The listing builds one solid part. Answer for the finished solid, in the listing's coordinates (mm). A direction names the side the tool comes from. Round coordinates to 2 decimals unless told otherwise and drop trailing zeros. Order: outer loops, then holes, each group sorted by start corner. A loop starts at its lowest first (then second) coordinate and runs counter-clockwise, first axis right, second up. Notation, with made-up numbers: M -5.5,-0.75 L 42.5,-0.75 A15 ccw 42.5,20.25 Z; hole C 16.5,7 d1. An arc over 180 degrees is marked long. Put each result on its own line as item: value. Start each with the question number.
1. The part is cut by section B-B (y = 28). Give the vertices of the cut face in (x, z).
2. The part is cut by section A-A (z = 2.25). Give the vertices of the cut face in (x, y), then the cut area to 3 significant figures.
3. The part is cut by section C-C (x = -28). Give the vertices of the cut face in (y, z).
4. The part is cut by section D-D (x = -52). Give the vertices of the cut face in (y, z).
5. The mould has two halves that part along Y. Classify faces 4 (the face through (-58, 22.298, 4)), 5 (the face through (-59, 28, 2.9)), 6 (the face through (-37, 33, 7.6)): +Y half, -Y half, draft (parallel to the pull), parting line (faces both ways), or undercut.
6. Consider line 1 (Y direction, x = -54, z = 4); line 2 (Z direction, x = -61, y = 33); line 3 (X direction, y = 30.5, z = 5.5). Determine where each line is inside the solid, lowest interval first.
7. Which of the six approach directions +Z, -Z, +X, -X, +Y, -Y give full straight-line access (tool end or side, diameter ignored) to faces 1 (the face through (-37, 26.648, 3)), 2 (the face through (-59, 33.498, 4)), 3 (the face through (-63, 25.848, 8))?
8. Each of these flat-tipped pins is pushed along its axis until it touches: pin 1 Ø0.9 at (y, z) = (27.5, 3.5) entering from -X; pin 2 Ø2.5 at (y, z) = (28.5, 3.5) entering from +X; pin 3 Ø7.5 at (x, y) = (-36.5, 32.5) entering from +Z. Where does it stop, or does it pass through?
from build123d import *

# Parameters (mm, degrees)
SKETCH1_W           = 39.5
SKETCH1_H           = 16.2
SKETCH1_R           = 1.5
BOSS_EXTRUDE1_DEPTH = 1.6
BOSS_EXTRUDE2_DEPTH = 6
SKETCH3_W           = 12.85
SKETCH3_H           = 3
CUT_EXTRUDE1_DEPTH  = 3
CUT_EXTRUDE3_DEPTH  = 3
SKETCH5_W           = 2.25
SKETCH5_H           = 2.25
CUT_EXTRUDE4_DEPTH  = 50.733422671
BOSS_EXTRUDE3_DEPTH = 6.75
CUT_EXTRUDE5_DEPTH  = 1.5
SKETCH8_W           = 2.65
SKETCH8_H           = 9.9
CUT_EXTRUDE6_DEPTH  = 12
CUT_EXTRUDE7_REACH  = 76.987
SKETCH9_W           = 0.35
SKETCH9_H           = 3
SKETCH9_W_2         = 0.175
BOSS_EXTRUDE4_DEPTH = 4.75
SKETCH11_W          = 12.85
SKETCH11_H          = 1.15
CUT_EXTRUDE8_DEPTH  = 4.75


with BuildPart() as part:
    # Sketch1 → Boss-Extrude1 (new body)
    with BuildSketch(Plane.XY):
        with Locations((-43.509331094, 28.548203647)):
            Rectangle(SKETCH1_W, SKETCH1_H)
        with Locations((-27.259331094, 33.648203647)):
            Circle(SKETCH1_R, mode=Mode.SUBTRACT)
        with Locations((-46.009331094, 33.648203647)):
            Circle(SKETCH1_R, mode=Mode.SUBTRACT)
    extrude(amount=BOSS_EXTRUDE1_DEPTH)

    # Sketch2 → Boss-Extrude2 (add)
    with BuildSketch(Plane.XY.offset(1.6)):
        Polygon((-30.509331094, 30.378901516), (-30.509331094, 36.648203647), (-43.359331094, 36.648203647), (-43.359331094, 26.648203647), (-30.509331094, 26.648203647), align=None)
    extrude(amount=BOSS_EXTRUDE2_DEPTH)

    # Sketch3 → Cut-Extrude1 (cut)
    with BuildSketch(Plane.XY.offset(7.6)):
        with Locations((-36.934331094, 28.148203647)):
            Rectangle(SKETCH3_W, SKETCH3_H)
    extrude(amount=-CUT_EXTRUDE1_DEPTH, mode=Mode.SUBTRACT)

    # Sketch4 → Cut-Extrude3 (cut)
    with BuildSketch(Plane.XY.offset(4.6)):
        Polygon((-32.509331094, 29.648203647), (-35.934331094, 29.648203647), (-35.934331094, 26.648203647), (-32.509331094, 26.648203647), (-32.509331094, 27.856511678), align=None)
        Polygon((-37.934331094, 29.648203647), (-41.359331094, 29.648203647), (-41.359331094, 28.148203647), (-41.359331094, 26.648203647), (-37.934331094, 26.648203647), align=None)
    extrude(amount=-CUT_EXTRUDE3_DEPTH, mode=Mode.SUBTRACT)

    # Sketch5 → Cut-Extrude4 (cut, through all)
    with BuildSketch(Plane(origin=(-30.509331094, 0, 0), x_dir=(0, 0, -1), z_dir=(1, 0, 0))):
        with Locations((-2.725, 28.523203647)):
            Rectangle(SKETCH5_W, SKETCH5_H)
    extrude(amount=-CUT_EXTRUDE4_DEPTH, mode=Mode.SUBTRACT)

    # Sketch6 → Boss-Extrude3 (add)
    with BuildSketch(Plane.XY.offset(1.6)):
        Polygon((-63.259331094, 22.298203647), (-63.259331094, 28.548203647), (-63.259331094, 34.798203647), (-65.259331094, 34.798203647), (-65.259331094, 22.298203647), align=None)
        Polygon((-63.259331094, 34.798203647), (-63.259331094, 28.548203647), (-63.259331094, 22.298203647), (-51.259331094, 22.298203647), (-51.259331094, 34.798203647), align=None)
    extrude(amount=BOSS_EXTRUDE3_DEPTH)

    # Sketch7 → Cut-Extrude5 (cut)
    with BuildSketch(Plane.XY.offset(8.35)):
        Polygon((-65.259331094, 34.798203647), (-65.259331094, 32.448203647), (-61.509331094, 32.448203647), (-61.509331094, 31.248203647), (-64.009331094, 31.248203647), (-64.009331094, 25.848203647), (-61.509331094, 25.848203647), (-61.509331094, 24.648203647), (-65.259331094, 24.648203647), (-65.259331094, 22.298203647), (-51.259331094, 22.298203647), (-51.259331094, 34.798203647), align=None)
    extrude(amount=-CUT_EXTRUDE5_DEPTH, mode=Mode.SUBTRACT)

    # Sketch8 → Cut-Extrude6 (cut)
    with BuildSketch(Plane.ZY.offset(65.259331094)):
        Polygon((6.85, 31.148203647), (5.55, 31.148203647), (5.55, 25.948203647), (6.85, 25.948203647), (7.6, 25.948203647), (7.6, 31.148203647), align=None)
        with Locations((4.225, 28.548203647)):
            Rectangle(SKETCH8_W, SKETCH8_H)
    extrude(amount=-CUT_EXTRUDE6_DEPTH, mode=Mode.SUBTRACT)

    # Cut-Extrude7: up to this face of the body (flat: up to its plane)
    cut_extrude7_end = Plane(part.part.faces().sort_by_distance((-39.983883979, 27.291998742, 1.6))[0])
    # Sketch9 → Cut-Extrude7 (cut, up to the picked face)
    with BuildSketch(Plane.XY.offset(4.6), mode=Mode.PRIVATE) as cut_extrude7_sk1:
        with Locations((-30.684331094, 28.148203647)):
            Rectangle(SKETCH9_W, SKETCH9_H)
    cut_extrude7_tool1 = split(extrude(cut_extrude7_sk1.sketch, amount=-CUT_EXTRUDE7_REACH, mode=Mode.PRIVATE), bisect_by=cut_extrude7_end, keep=Keep.BOTH, mode=Mode.PRIVATE)
    # Sketch9 → Cut-Extrude7 (cut, up to the picked face)
    with BuildSketch(Plane.XY.offset(4.6), mode=Mode.PRIVATE) as cut_extrude7_sk2:
        with Locations((-43.184331094, 28.148203647)):
            Rectangle(SKETCH9_W, SKETCH9_H)
    cut_extrude7_tool2 = split(extrude(cut_extrude7_sk2.sketch, amount=-CUT_EXTRUDE7_REACH, mode=Mode.PRIVATE), bisect_by=cut_extrude7_end, keep=Keep.BOTH, mode=Mode.PRIVATE)
    # Sketch9 → Cut-Extrude7 (cut, up to the picked face)
    with BuildSketch(Plane.XY.offset(4.6), mode=Mode.PRIVATE) as cut_extrude7_sk3:
        with Locations((-37.846831094, 28.148203647)):
            Rectangle(SKETCH9_W_2, SKETCH9_H)
    cut_extrude7_tool3 = split(extrude(cut_extrude7_sk3.sketch, amount=-CUT_EXTRUDE7_REACH, mode=Mode.PRIVATE), bisect_by=cut_extrude7_end, keep=Keep.BOTH, mode=Mode.PRIVATE)
    # Sketch9 → Cut-Extrude7 (cut, up to the picked face)
    with BuildSketch(Plane.XY.offset(4.6), mode=Mode.PRIVATE) as cut_extrude7_sk4:
        with Locations((-36.021831094, 28.148203647)):
            Rectangle(SKETCH9_W_2, SKETCH9_H)
    cut_extrude7_tool4 = split(extrude(cut_extrude7_sk4.sketch, amount=-CUT_EXTRUDE7_REACH, mode=Mode.PRIVATE), bisect_by=cut_extrude7_end, keep=Keep.BOTH, mode=Mode.PRIVATE)
    add(cut_extrude7_tool1.solids().sort_by(Axis((-30.684331, 28.148204, 4.6), (0, 0, -1)))[0], mode=Mode.SUBTRACT)
    add(cut_extrude7_tool2.solids().sort_by(Axis((-43.184331, 28.148204, 4.6), (0, 0, -1)))[0], mode=Mode.SUBTRACT)
    add(cut_extrude7_tool3.solids().sort_by(Axis((-37.846831, 28.148204, 4.6), (0, 0, -1)))[0], mode=Mode.SUBTRACT)
    add(cut_extrude7_tool4.solids().sort_by(Axis((-36.021831, 28.148204, 4.6), (0, 0, -1)))[0], mode=Mode.SUBTRACT)

    # Sketch10 → Boss-Extrude4 (add)
    with BuildSketch(Plane.XY.offset(7.6)):
        Polygon((-30.509331094, 40.033691869), (-43.359331094, 36.648203647), (-42.954120568, 36.648203647), (-30.509331094, 39.809326044), align=None)
    extrude(amount=-BOSS_EXTRUDE4_DEPTH)

    # Sketch11 → Cut-Extrude8 (cut)
    with BuildSketch(Plane(origin=(0, 36.648203647, 0), x_dir=(1, 0, 0), z_dir=(0, 1, 0))):
        with Locations((-36.934331094, -7.025)):
            Rectangle(SKETCH11_W, SKETCH11_H)
    extrude(amount=CUT_EXTRUDE8_DEPTH, mode=Mode.SUBTRACT)


solid = part.part
Resolved:
1. outline: M -65.26,1.6 L -63.26,1.6 L -63.26,0 L -23.76,0 L -23.76,1.6 L -51.26,1.6 L -51.26,6.85 L -53.26,6.85 L -53.26,2.9 L -65.26,2.9 Z; M -65.26,7.6 L -64.01,7.6 L -64.01,8.35 L -65.26,8.35 Z; M -43.01,3.85 L -41.36,3.85 L -41.36,4.6 L -43.01,4.6 Z; M -37.76,3.85 L -36.11,3.85 L -36.11,4.6 L -37.76,4.6 Z; M -32.51,3.85 L -30.86,3.85 L -30.86,4.6 L -32.51,4.6 Z
2. outline: M -65.26,22.3 L -51.26,22.3 L -51.26,34.8 L -65.26,34.8 Z; M -43.36,29.65 L -30.51,29.65 L -30.51,36.65 L -43.36,36.65 Z; M -43.01,26.65 L -41.36,26.65 L -41.36,27.4 L -43.01,27.4 Z; M -37.76,26.65 L -36.11,26.65 L -36.11,27.4 L -37.76,27.4 Z; M -32.51,26.65 L -30.86,26.65 L -30.86,27.4 L -32.51,27.4 Z
2. area: 269 mm2
3. outline: M 20.45,0 L 32.34,0 L 32.34,1.6 L 20.45,1.6 Z; M 34.95,0 L 36.65,0 L 36.65,1.6 L 34.95,1.6 Z
4. outline: M 20.45,0 L 36.65,0 L 36.65,1.6 L 34.8,1.6 L 34.8,6.85 L 22.3,6.85 L 22.3,1.6 L 20.45,1.6 Z
5. face 4: -Y half
5. face 5: undercut
5. face 6: draft
6. line 1: 22.3 to 23.6, 33.5 to 34.8
6. line 2: 0 to 2.9, 5.55 to 6.85
6. line 3: -53.26 to -51.26, -43.36 to -30.51
7. face 1: +Z, +X, -Y
7. face 2: -X
7. face 3: +Z, +X
8. pin 1: x = -53.26
8. pin 2: x = -30.51
8. pin 3: z = 7.6
